```python
from build123d import *

# Parameters (mm, degrees)
SKETCH1_R           = 4.627548386
SKETCH1_R_2         = 1
BOSS_EXTRUDE1_DEPTH = 4
BOSS_EXTRUDE3_DEPTH = 2
SKETCH5_W           = 4.5
SKETCH5_H           = 3.78546494
BOSS_EXTRUDE4_DEPTH = 1
CUT_EXTRUDE1_DEPTH  = 47.280842529
D_GAGEMENT_M31_D    = 3.4


with BuildPart() as part:
    # Sketch1 → Boss-Extrude1 (new body)
    # profile 1 of 9: a face of its own
    with BuildSketch(Plane.XY):
        with BuildLine():
            Line((-6, 44), (-14, 44))
            Line((-14, 44), (-14, 26))
            Line((-14, 26), (-10, 26))
            ThreePointArc((-10, 26), (-4, 20), (-10, 14))
            Line((-10, 14), (-14, 14))
            Line((-14, 14), (-14, -4))
            Line((-14, -4), (-6, -4))
            Line((-6, -4), (-6, 0))
            ThreePointArc((-6, 0), (0, 6), (6, 0))
            Line((6, 0), (6, -4))
            Line((6, -4), (14, -4))
            Line((14, -4), (14, 14))
            Line((14, 14), (10, 14))
            ThreePointArc((10, 14), (4, 20), (10, 26))
            Line((10, 26), (14, 26))
            Line((14, 26), (14, 44))
            Line((14, 44), (6, 44))
            Line((6, 44), (6, 40))
            ThreePointArc((6, 40), (0, 34), (-6, 40))
            Line((-6, 40), (-6, 44))
        make_face()
        with Locations((0, 12.3952)):
            Circle(SKETCH1_R, mode=Mode.SUBTRACT)
        with Locations((-10, 30)):
            Circle(SKETCH1_R_2, mode=Mode.SUBTRACT)
        with Locations((10, 30)):
            Circle(SKETCH1_R_2, mode=Mode.SUBTRACT)
    # profile 2 of 9: a face of its own
    with BuildSketch(Plane.XY):
        with BuildLine():
            Line((-14, 14), (-14, 26))
            Line((-14, 26), (-18, 26))
            ThreePointArc((-18, 26), (-24, 20), (-18, 14))
            Line((-18, 14), (-14, 14))
        make_face()
    # profile 3 of 9: a face of its own
    with BuildSketch(Plane.XY):
        with BuildLine():
            Line((-10, 26), (-14, 26))
            Line((-14, 26), (-14, 14))
            Line((-14, 14), (-10, 14))
            ThreePointArc((-10, 14), (-4, 20), (-10, 26))
        make_face()
    # profile 4 of 9: a face of its own
    with BuildSketch(Plane.XY):
        with BuildLine():
            Line((6, 44), (-6, 44))
            Line((-6, 44), (-6, 40))
            ThreePointArc((-6, 40), (0, 34), (6, 40))
            Line((6, 40), (6, 44))
        make_face()
    # profile 5 of 9: a face of its own
    with BuildSketch(Plane.XY):
        with BuildLine():
            Line((-6, 48), (-6, 44))
            Line((-6, 44), (6, 44))
            Line((6, 44), (6, 48))
            ThreePointArc((6, 48), (0, 54), (-6, 48))
        make_face()
    # profile 6 of 9: a face of its own
    with BuildSketch(Plane.XY):
        with BuildLine():
            Line((14, 14), (14, 26))
            Line((14, 26), (10, 26))
            ThreePointArc((10, 26), (4, 20), (10, 14))
            Line((10, 14), (14, 14))
        make_face()
    # profile 7 of 9: a face of its own
    with BuildSketch(Plane.XY):
        with BuildLine():
            Line((18, 26), (14, 26))
            Line((14, 26), (14, 14))
            Line((14, 14), (18, 14))
            ThreePointArc((18, 14), (24, 20), (18, 26))
        make_face()
    # profile 8 of 9: a face of its own
    with BuildSketch(Plane.XY):
        with BuildLine():
            Line((-6, 0), (-6, -4))
            Line((-6, -4), (6, -4))
            Line((6, -4), (6, 0))
            ThreePointArc((6, 0), (0, 6), (-6, 0))
        make_face()
        Circle(SKETCH1_R_2, mode=Mode.SUBTRACT)
    # profile 9 of 9: a face of its own
    with BuildSketch(Plane.XY):
        with BuildLine():
            Line((6, -4), (-6, -4))
            Line((-6, -4), (-6, -8))
            ThreePointArc((-6, -8), (0, -14), (6, -8))
            Line((6, -8), (6, -4))
        make_face()
    extrude(amount=BOSS_EXTRUDE1_DEPTH)

    # Sketch4 → Boss-Extrude3 (add)
    with BuildSketch(Plane(origin=(0, 0, 0), x_dir=(-1, 0, 0), z_dir=(0, 0, -1))):
        Polygon((-6, 44), (-14, 44), (-14, 26), (-14, 14), (-14, -4), (-6, -4), (6, -4), (14, -4), (14, 14), (14, 26), (14, 44), (6, 44), align=None)
        with BuildLine():
            Line((-10.5, 32.449489743), (-10.5, 40.5))
            Line((-10.5, 40.5), (10.5, 40.5))
            Line((10.5, 40.5), (10.5, 32.449489743))
            ThreePointArc((10.5, 32.449489743), (11.936491673, 31.58113883), (12.5, 30))
            ThreePointArc((12.5, 30), (11.936491673, 28.41886117), (10.5, 27.550510257))
            Line((10.5, 27.550510257), (10.5, -0.5))
            Line((10.5, -0.5), (2.449489743, -0.5))
            ThreePointArc((2.449489743, -0.5), (0, -2.5), (-2.449489743, -0.5))
            Line((-2.449489743, -0.5), (-10.5, -0.5))
            Line((-10.5, -0.5), (-10.5, 27.550510257))
            ThreePointArc((-10.5, 27.550510257), (-12.5, 30), (-10.5, 32.449489743))
        make_face(mode=Mode.SUBTRACT)
    extrude(amount=BOSS_EXTRUDE3_DEPTH)

    # Sketch5 → Boss-Extrude4 (add)
    with BuildSketch(Plane(origin=(0, 0, -2), x_dir=(-1, 0, 0), z_dir=(0, 0, -1))):
        with Locations((-11.75, 23.476244976)):
            Rectangle(SKETCH5_W, SKETCH5_H)
        with Locations((11.75, 23.476244976)):
            Rectangle(SKETCH5_W, SKETCH5_H)
    extrude(amount=BOSS_EXTRUDE4_DEPTH)

    # Sketch7 → Cut-Extrude1 (cut, through all)
    with BuildSketch(Plane(origin=(0, 25.368977446, 0), x_dir=(1, 0, 0), z_dir=(0, 1, 0))):
        Polygon((-10.5, 2), (-9.5, 3), (-9.5, 2), align=None)
        Polygon((10.5, 2), (9.5, 3), (9.5, 2), align=None)
    extrude(amount=-CUT_EXTRUDE1_DEPTH, mode=Mode.SUBTRACT)

    # Dégagement M31 (through all)
    with Locations(Plane.XY.offset(4)):
        with Locations((0, 48), (0, -8), (-18, 20), (18, 20)):
            Hole(D_GAGEMENT_M31_D / 2)


solid = part.part
```
The model under review builds one solid part; all positions refer to its coordinate system, in mm. A direction names the side the tool comes from. Give positions to 0.01 mm unless a question says otherwise; leave off trailing zeros. Loops run counter-clockwise (first coordinate to the right, second up) from the corner with the lowest first, then second, coordinate; pieces in that order, holes last. Notation, with made-up numbers: (40.5, 36) -> (65.5, 36) arc R28 cw to (65.5, 69) -> close; hole circle Ø5 at (-12, -20.5). An arc over 180 degrees is marked (long way). Use CSV: the item, a comma, the result in double quotes.
1. Consider section B-B, the plane z = -1.25. Write out the cut boundary in (x, y), then the cut area to 3 significant figures.
Result:
outline,"(-14, -4) -> (14, -4) -> (14, 44) -> (-14, 44) -> close; hole (-10.5, -0.5) -> (-2.45, -0.5) arc R2.5 ccw to (2.45, -0.5) -> (10.5, -0.5) -> (10.5, 27.55) arc R2.5 ccw to (10.5, 32.45) -> (10.5, 40.5) -> (-10.5, 40.5) -> (-10.5, 32.45) arc R2.5 ccw to (-10.5, 27.55) -> close"
area,"461 mm²"
2. The part is to be moulded in two halves that separate along Y. For faces 5 (the face through (20, 20, 0)), 6 (the face through (-16, 26, 2)), 7 (the face through (0, -14, 2)), 8 (the face through (0, 19, 0)), say which applies: +Y half, -Y half, draft (parallel to the pull), parting line (faces both ways), or undercut.
Result:
face 5,"draft"
face 6,"+Y half"
face 7,"-Y half"
face 8,"undercut"
3. For P1, Ø1.2, axis at x = -16.5, z = 2, coming from the -Y side; P2, Ø0.8, axis at x = 11, z = -2.5, coming from the +Y side; P3, Ø2, axis at y = 47, z = 1.5, coming from the +X side, all flat-tipped, find the tip position at first contact; note any pin that passes through.
Result:
P1,"stops at y = 14"
P2,"stops at y = 25.37"
P3,"stops at x = 6"
4. To check wall thickness, follow probe 1 along Y at (x, z) = (0, 2.45); probe 2 along Y at (x, z) = (0.5, -0.5); probe 3 along Y at (x, z) = (-7, -1.5). State the ranges of each line that lie inside material, in increasing order. Write a range as from..to.
Result:
probe 1,"y = -14..-9.7, -6.3..-1, 1..7.77, 17.02..46.3, 49.7..54"
probe 2,"y = -4..-2.45, 40.5..44"
probe 3,"y = -4..-0.5, 40.5..44"
5. Machinability: for faces 1 (the face through (-7, -0.5, -1)), 2 (the face through (-6, -6, 2)), 3 (the face through (0, 50, 0)), 4 (the face through (0, -10, 0)), which of the approach directions +Z, -Z, +X, -X, +Y, -Y give a long, thin tool a straight path to every point of the face, cutting with its end or side? Answer none if there is none.
Result:
face 1,"-Z"
face 2,"+Z, -Z, -X, -Y"
face 3,"-Z, +X, -X, +Y"
face 4,"-Z, +X, -X, -Y"
6. Consider section D-D, the plane y = 39. Write out the cut boundary in (x, z), then the cut area to 3 significant figures.
Result:
outline,"(-14, -2) -> (-10.5, -2) -> (-10.5, 0) -> (10.5, 0) -> (10.5, -2) -> (14, -2) -> (14, 4) -> (-14, 4) -> close"
area,"126 mm²"
7. Consider section A-A, the plane y = 20. Write out the cut boundary in (x, z), then the cut area to 3 significant figures.
Result:
outline,"(-24, 0) -> (-19.7, 0) -> (-19.7, 4) -> (-24, 4) -> close; (-16.3, 0) -> (-14, 0) -> (-14, -2) -> (-10.5, -2) -> (-10.5, 0) -> (10.5, 0) -> (10.5, -2) -> (14, -2) -> (14, 0) -> (16.3, 0) -> (16.3, 4) -> (-16.3, 4) -> close; (19.7, 0) -> (24, 0) -> (24, 4) -> (19.7, 4) -> close"
area,"179 mm²"
8. Consider section C-C, the plane x = 3.5. Write out the cut boundary in (y, z).
Result:
outline,"(-12.87, 0) -> (-4, 0) -> (-4, -2) -> (-0.5, -2) -> (-0.5, 0) -> (9.37, 0) -> (9.37, 4) -> (-12.87, 4) -> close; (15.42, 0) -> (40.5, 0) -> (40.5, -2) -> (44, -2) -> (44, 0) -> (52.87, 0) -> (52.87, 4) -> (15.42, 4) -> close"
